from build123d import *

# Parameters (mm, degrees)
SKETCH1_R           = 102.87
SKETCH1_R_2         = 6.35
BOSS_EXTRUDE1_DEPTH = 6.35
SKETCH6_R           = 20.32
CUT_EXTRUDE1_DEPTH  = 28.448


with BuildPart() as part:
    # Sketch1 → Boss-Extrude1 (new body)
    with BuildSketch(Plane(origin=(0, 0, 0), x_dir=(1, 0, 0), z_dir=(0, 1, 0))):
        with BuildLine():
            Line((256.521079071, 133.368920929), (0, 133.368920929))
            ThreePointArc((0, 133.368920929), (-94.306068389, 94.306068389), (-133.368920929, 0))
            Line((-133.368920929, 0), (-133.368920929, -95.231079071))
            ThreePointArc((-133.368920929, -95.231079071), (-129.64917705, -104.211335192), (-120.668920929, -107.931079071))
            Line((-120.668920929, -107.931079071), (227.955539535, -107.931079071))
            ThreePointArc((227.955539535, -107.931079071), (230.193914007, -107.003914007), (231.121079071, -104.765539535))
            Line((231.121079071, -104.765539535), (231.121079071, 3.100777109))
            ThreePointArc((231.121079071, 3.100777109), (232.98095101, 7.59090517), (237.471079071, 9.450777109))
            Line((237.471079071, 9.450777109), (256.521079071, 9.450777109))
            ThreePointArc((256.521079071, 9.450777109), (261.011207131, 11.310649048), (262.871079071, 15.800777109))
            Line((262.871079071, 15.800777109), (262.871079071, 127.018920929))
            ThreePointArc((262.871079071, 127.018920929), (261.011207131, 131.50904899), (256.521079071, 133.368920929))
        make_face()
        Circle(SKETCH1_R, mode=Mode.SUBTRACT)
        with Locations((-112.738641363, -14.374963544)):
            Circle(SKETCH1_R_2, mode=Mode.SUBTRACT)
        with Locations((43.920237074, 104.822009181)):
            Circle(SKETCH1_R_2, mode=Mode.SUBTRACT)
        with Locations((68.818404289, -90.447045637)):
            Circle(SKETCH1_R_2, mode=Mode.SUBTRACT)
        with Locations((250.171079071, 107.968920929)):
            Circle(SKETCH1_R_2, mode=Mode.SUBTRACT)
        with Locations((250.171079071, 34.850777109)):
            Circle(SKETCH1_R_2, mode=Mode.SUBTRACT)
    extrude(amount=BOSS_EXTRUDE1_DEPTH)

    # Sketch6 → Cut-Extrude1 (cut)
    with BuildSketch(Plane(origin=(0, 0, 0), x_dir=(1, 0, 0), z_dir=(0, 1, 0))):
        with Locations((174.732998702, 0.124686489)):
            Circle(SKETCH6_R)
    extrude(amount=CUT_EXTRUDE1_DEPTH, mode=Mode.SUBTRACT)


solid = part.part
Design review of the part built by this model. Coordinates are the model's own, in mm. Round coordinates to 2 decimals unless told otherwise and drop trailing zeros. Order: outer loops, then holes, each group sorted by start corner. A loop starts at its lowest first (then second) coordinate and runs counter-clockwise, first axis right, second up. Notation, with made-up numbers: M 42,77.25 L 58,77.25 A22 cw 58,83.25 Z; hole C 63,47 d1. An arc over 180 degrees is marked long. Answer as CSV lines item,"result". Start each with the question number.
1) The part is to be moulded in two halves that separate along Z. For faces 1 (the face through (-93.3, 3.1, -95.3)), 2 (the face through (-109.325, 3.131, 9.021)), 3 (the face through (106, 0, -14)), say which applies: +Z half, -Z half, draft (parallel to the pull), parting line (faces both ways), or undercut.
2) For pin 1 Ø16.5 at (x, z) = (-112.74, 14.37) entering from +Y; pin 2 Ø1.9 at (x, y) = (248.5, 3) entering from +Z, all flat-tipped, find the tip position at first contact; note any pin that passes through.
3) Wall thickness on line 1 along X through (y, z) = (4, 0); line 2 along Z through (x, y) = (3, 2.25); line 3 along X through (y, z) = (2, 9): over which ranges is each line inside the solid? List them lowest first. Write a range as [from, to].
4) Add section C-C (y = 4.75). Give the boundary of the cut face in (x, z).
5) Add section B-B (z = 43.5). Give the boundary of the cut face in (x, y).
6) Add section A-A (x = 32). Give the boundary of the cut face in (y, z).
Resolved:
1,face 1,"-Z half"
1,face 2,"undercut"
1,face 3,"draft"
2,pin 1,"y = 6.35"
2,pin 2,"z = -9.45"
3,line 1,"[-133.37, -102.87], [102.87, 154.41], [195.05, 231.12]"
3,line 2,"[-133.37, -102.83], [102.83, 107.93]"
3,line 3,"[-133.37, -116.12], [-109.36, -102.48], [102.48, 156.58], [192.89, 231.12]"
4,outline,"M -133.37,0 A133.37 ccw 0,-133.37 L 256.52,-133.37 A6.35 ccw 262.87,-127.02 L 262.87,-15.8 A6.35 ccw 256.52,-9.45 L 237.47,-9.45 A6.35 cw 231.12,-3.1 L 231.12,104.77 A3.17 ccw 227.96,107.93 L -120.67,107.93 A12.7 ccw -133.37,95.23 Z; hole C -112.74,14.37 d12.7; hole C 0,0 d205.74; hole C 43.92,-104.82 d12.7; hole C 68.82,90.45 d12.7; hole C 174.73,-0.12 d40.64; hole C 250.17,-107.97 d12.7; hole C 250.17,-34.85 d12.7"
5,outline,"M -133.37,0 L -93.22,0 L -93.22,6.35 L -133.37,6.35 Z; M 93.22,0 L 231.12,0 L 231.12,6.35 L 93.22,6.35 Z"
6,outline,"M 0,-133.37 L 6.35,-133.37 L 6.35,-97.77 L 0,-97.77 Z; M 0,97.77 L 6.35,97.77 L 6.35,107.93 L 0,107.93 Z"
